The drawing under review shows one solid part. Ordinate dimensions are in mm from its lowest x, y, z. A direction names the side the tool comes from. Round coordinates to 2 decimals unless told otherwise and drop trailing zeros. Loops run counter-clockwise (first coordinate to the right, second up) from the corner with the lowest first, then second, coordinate; pieces in that order, holes last. Notation, with made-up numbers: (-24, 74) - (16, 74) arc R16 cw to (16, 81) - close; hole circle Ø5 at (81, 84). An arc over 180 degrees is marked (long way). Answer as CSV lines item,"result".
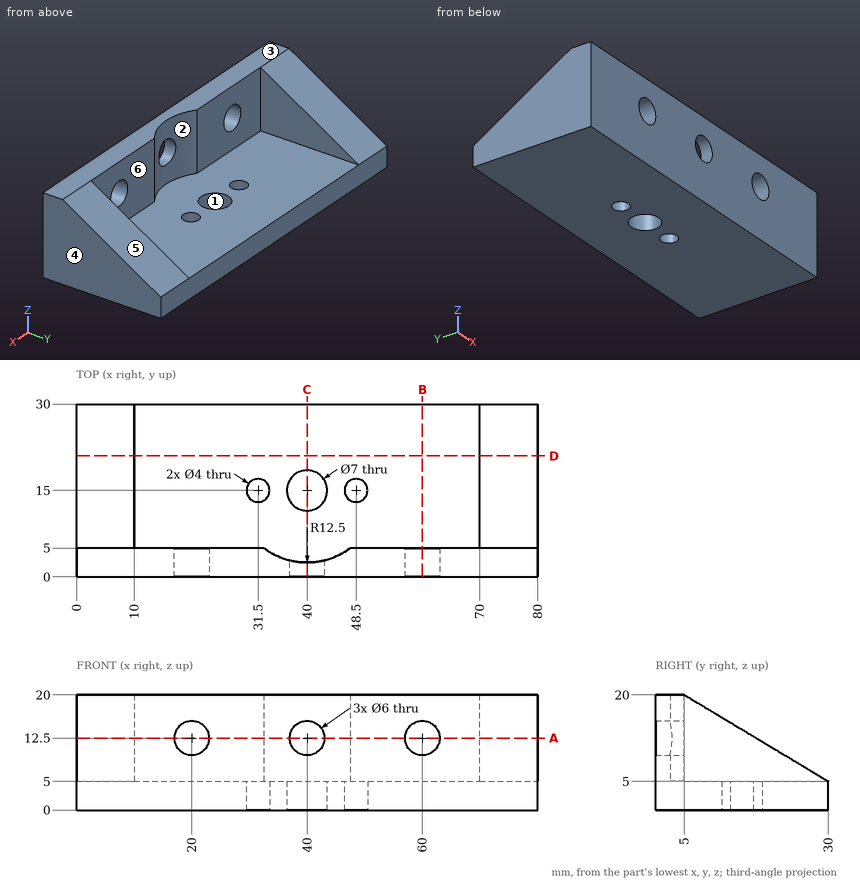
1. Take a section at D-D (y = 21). State the section outline as (x, z) points, plus the area to 3 significant figures.
Numbers:
outline,"(0, 0) - (80, 0) - (80, 10.4) - (70, 10.4) - (70, 5) - (10, 5) - (10, 10.4) - (0, 10.4) - close"
area,"508 mm²"
2. Draft analysis for pull direction X (two halves, no side actions). For the marked faces 1, 2, 3 and 4, state which applies: +X half, -X half, draft (parallel to the pull), parting line (faces both ways), or undercut.
Numbers:
face 1,"undercut"
face 2,"undercut"
face 3,"draft"
face 4,"+X half"
3. Tool access review of the marked faces 5 and 6: name each direction out of +Z, -Z, +X, -X, +Y, -Y from which nothing blocks a thin tool from reaching the whole face with its end or side.
Numbers:
face 5,"+Z, +X, -X, +Y"
face 6,"+Z, +Y"
4. Take a section at A-A (z = 12.5). State the section outline as (x, y) points.
Numbers:
outline,"(0, 0) - (17, 0) - (17, 5) - (10, 5) - (10, 17.5) - (0, 17.5) - close; (23, 0) - (37, 0) - (37, 2.87) arc R12.5 cw to (32.5, 5) - (23, 5) - close; (43, 0) - (57, 0) - (57, 5) - (47.5, 5) arc R12.5 cw to (43, 2.87) - close; (63, 0) - (80, 0) - (80, 17.5) - (70, 17.5) - (70, 5) - (63, 5) - close"
5. Take a section at C-C (x = 40). State the section outline as (y, z) points, plus the area to 4 significant figures.
Numbers:
outline,"(0, 0) - (11.5, 0) - (11.5, 5) - (2.5, 5) - (2.5, 9.5) - (0, 9.5) - close; (0, 15.5) - (2.5, 15.5) - (2.5, 20) - (0, 20) - close; (18.5, 0) - (30, 0) - (30, 5) - (18.5, 5) - close"
area,"137.5 mm²"
6. Wall thickness on probe 1 along Z at (x, y) = (20, 3.7); probe 2 along Y at (x, z) = (31.5, 2.85); probe 3 along X at (y, z) = (20.5, 7.5): over which ranges is each line inside the solid? List them lowest first.
Numbers:
probe 1,"z = 0 to 9.5, 15.5 to 20"
probe 2,"y = 0 to 13, 17 to 30"
probe 3,"x = 0 to 10, 70 to 80"
7. Clearance check with flat-ended pins moving along their axes: pin 1 (3 mm diameter, centred on x = 54, y = 21.5, fed in from +Z); pin 2 (6 mm diameter, centred on x = 10.5, y = 10, fed in from +Z); pin 3 (4.5 mm diameter, centred on x = 55.5, z = 10.5, fed in from +Y). State where each tip first meets the part, or that it passes through.
Numbers:
pin 1,"stops at z = 5"
pin 2,"stops at z = 18.77"
pin 3,"stops at y = 5"
8. Take a section at B-B (x = 60). State the section outline as (y, z) points.
Numbers:
outline,"(0, 0) - (30, 0) - (30, 5) - (5, 5) - (5, 9.5) - (0, 9.5) - close; (0, 15.5) - (5, 15.5) - (5, 20) - (0, 20) - close"
